from build123d import *

# Parameters (mm, degrees)
F0_R            = 53.8517918496
F1_DEPTH        = 12.7
F3_DEPTH        = 25.4
F3_COPIES_COUNT = 20
F5_DEPTH        = 12.7
F5_COPIES_COUNT = 8
F7_DEPTH        = 12.7
F7_COPIES_COUNT = 4


# Not quite as in the source:
# - a pattern or mirror of a feature is missing from the dataset's text; its kind, count and spacing are read off the source's solid


with BuildPart() as f1:
    # F0 (on Front) → F1 (new body, symmetric)
    with BuildSketch(Plane.XZ):
        Circle(F0_R)
    extrude(amount=F1_DEPTH, both=True)

    # F2 (on face) → F3 (join, through all)
    with BuildSketch(Plane.XZ.offset(12.7)):
        Polygon((17.4729507416, -58.154836297), (17.9823680134, -50.7607124264), (5.4343099044, -53.5768957786), (10.3754857555, -60.3680238128), (13.1992083043, -56.0942813754), align=None)
    f3 = extrude(amount=-F3_DEPTH)

    # F3_copies: F3 ×20 about axis
    f3_copies_axis = Axis((0, 0, 0), (0, 1, 0))
    for i in range(1, F3_COPIES_COUNT):
        add(f3.rotate(f3_copies_axis, i * 360 / F3_COPIES_COUNT))

    # F4 (on face) → F5 (join)
    with BuildSketch(Plane(origin=(0, 12.7, 0), x_dir=(-1, 0, 0), z_dir=(0, 1, 0))):
        Polygon((32.4746519327, -31.217938289), (32.0429392159, -25.8215237409), (37.223495543, -25.8215237409), (32.9063646495, -20.5330364406), (25.2434555441, -28.7355873734), align=None)
    f5 = extrude(amount=F5_DEPTH)

    # F5_copies: F5 ×8 about axis
    f5_copies_axis = Axis((0, 0, 0), (0, 1, 0))
    for i in range(1, F5_COPIES_COUNT):
        add(f5.rotate(f5_copies_axis, i * 360 / F5_COPIES_COUNT))

    # F6 (on face) → F7 (join)
    with BuildSketch(Plane(origin=(0, 12.7, 0), x_dir=(-1, 0, 0), z_dir=(0, 1, 0))):
        Polygon((-18.7933090678, 14.4219585457), (-26.7386548221, 15.6052242965), (-29.1993897408, 5.2935681306), (-20.8797585219, 5.2935681306), (-24.5122741908, 10.0978622213), align=None)
    f7 = extrude(amount=F7_DEPTH)

    # F7_copies: F7 ×4 about axis
    f7_copies_axis = Axis((0, 0, 0), (0, 1, 0))
    for i in range(1, F7_COPIES_COUNT):
        add(f7.rotate(f7_copies_axis, i * 360 / F7_COPIES_COUNT))


solid = f1.part
Model file for the job. Use its own axes, mm. A direction names the side the tool comes from. Give positions to 0.01 mm unless a question says otherwise; leave off trailing zeros. Put each result on its own line as item: value. Start each with the question number.
(1) Tool access for faces 4 (the face through (15.31, -0.18, -57.11)), 5 (the face through (7.7, 19, -22.7)), 6 (the face through (15.005, 18.961, -22.71)), 7 (the face through (-23.214, 18.961, 35.095)), 8 (the face through (-33.7, -0.18, 46.36)): list every direction of +Z, -Z, +X, -X, +Y, -Y with a clear straight run to the whole face (end or side of a thin tool).
(2) Drill centre lines: L1, parallel to Z at x = -21, y = 17; L2, parallel to Y at x = 13.5, z = -15.5; L3, parallel to X at y = 23, z = -23.5. Where is each one in solid material? Low to high. Write a range as [from, to].
(3) Band-saw the part on A-A on y = 16.5. Count the separate pieces of the cut face and the enclosed holes in it, then the cut area to 3 significant figures.
(4) Pull direction Z, two halves, no side cores. Call faces 1 (the face through (35.095, 18.961, 23.214)), 2 (the face through (51.71, -0.18, 25.08)), 3 (the face through (-10.522, 18.961, 27.952)): released by +Z, released by -Z, zero draft, split by the parting line, or undercut.
(5) Pin check, flat tips, straight feed: pin 1 Ø2.5 at (y, z) = (21.5, 35) entering from -X; pin 2 Ø1.5 at (y, z) = (-2.5, 28.5) entering from +X; pin 3 Ø4 at (y, z) = (14, -36.5) entering from -X. Stop position of each tip, or through.
Results below:
1. face 4: -Z, +Y, -Y
1. face 5: +Y
1. face 6: +Z, +Y
1. face 7: +Z, +X, +Y
1. face 8: -X, +Y, -Y
2. L1: z = [-14.75, -12.75], [-5.45, -5.29], [32.47, 33.29]
2. L2: y = [-12.7, 12.7]
2. L3: x = [-35.33, -30.13], [5.29, 8.76], [10.86, 15.12]
3. separate pieces: 12
3. enclosed holes: 0
3. area: 630 mm2
4. face 1: released by -Z
4. face 2: undercut
4. face 3: released by +Z
5. pin 1: stops at x = -25.82
5. pin 2: stops at x = 54.21
5. pin 3: stops at x = -40.94
